Work out the finished part from the listing and answer in its coordinate system (mm). A direction names the side the tool comes from. Round coordinates to 2 decimals unless told otherwise and drop trailing zeros. Write each loop counter-clockwise with the first axis right and the second up, starting at its lowest first coordinate (ties: lowest second). Pieces come first, ordered by that corner, then holes. Notation, with made-up numbers: (89, 2) -> (105, 2) arc R9 ccw to (105, 9) -> close; hole circle Ø8 at (-10.5, 55.25). An arc over 180 degrees is marked (long way). Answer as a JSON object with one key per item and string values. Group by question number.
from build123d import *

# Parameters (mm, degrees)
SALIENTE_EXTRUIR1_DEPTH = 3.3


with BuildPart() as part:
    # Croquis1 → Saliente-Extruir1 (new body)
    with BuildSketch(Plane.XY):
        with BuildLine():
            Line((1.7, 25.8), (1.7, 35.8))
            ThreePointArc((1.7, 35.8), (4.712607831, 36.376098873), (7.730904305, 36.921609869))
            Line((7.730904305, 36.921609869), (7.730904305, 48.38))
            Line((7.730904305, 48.38), (1.7, 48.38))
            Line((1.7, 48.38), (-3.3, 48.38))
            Line((-3.3, 48.38), (-3.3, 58.38))
            Line((-3.3, 58.38), (0, 58.38))
            ThreePointArc((0, 58.38), (60, 62.669337163), (120, 58.38))
            Line((120, 58.38), (123.3, 58.38))
            Line((123.3, 58.38), (123.3, 48.38))
            Line((123.3, 48.38), (118.3, 48.38))
            Line((118.3, 48.38), (112.269095695, 48.38))
            Line((112.269095695, 48.38), (112.269095695, 36.921609869))
            ThreePointArc((112.269095695, 36.921609869), (115.287392169, 36.376098873), (118.3, 35.8))
            Line((118.3, 35.8), (118.3, 25.8))
            Line((118.3, 25.8), (123.3, 25.8))
            Line((123.3, 25.8), (123.3, 0))
            Line((123.3, 0), (120, 0))
            ThreePointArc((120, 0), (60, 35.797503597), (0, 0))
            Line((0, 0), (-3.3, 0))
            Line((-3.3, 0), (-3.3, 25.8))
            Line((-3.3, 25.8), (1.7, 25.8))
        make_face()
        with BuildLine():
            Line((17.730904305, 48.38), (17.730904305, 38.504540112))
            ThreePointArc((17.730904305, 38.504540112), (26.351558557, 39.595469902), (35, 40.438243974))
            Line((35, 40.438243974), (35, 48.38))
            Line((35, 48.38), (17.730904305, 48.38))
        make_face(mode=Mode.SUBTRACT)
        with BuildLine():
            Line((45, 48.38), (45, 41.101210552))
            ThreePointArc((45, 41.101210552), (60, 41.473490482), (75, 41.101210552))
            Line((75, 41.101210552), (75, 48.38))
            Line((75, 48.38), (45, 48.38))
        make_face(mode=Mode.SUBTRACT)
        with BuildLine():
            Line((85, 40.438243974), (85, 48.38))
            Line((85, 48.38), (102.269095695, 48.38))
            Line((102.269095695, 48.38), (102.269095695, 38.504540112))
            ThreePointArc((102.269095695, 38.504540112), (93.648441443, 39.595469902), (85, 40.438243974))
        make_face(mode=Mode.SUBTRACT)
    extrude(amount=SALIENTE_EXTRUIR1_DEPTH)


solid = part.part
1) A cutting plane is placed at B-B on z = 0.75. State how many separate pieces and enclosed holes the cut face has, plus the area to 3 significant figures.
2) A cutting plane is placed at A-A on x = 64. Determine the outline of the cut face in (y, z), plus the area to 3 significant figures.
3) Each of these flat-tipped pins is pushed along its axis until it touches: P1, Ø1.6, axis at y = 44, z = 1, coming from the +X side; P2, Ø1.6, axis at x = 92.5, z = 1.5, coming from the -Y side; P3, Ø1.5, axis at y = 35.5, z = 1.5, coming from the -X side. Where does it stop, or does it pass through?
4) A tool of negligible diameter and unlimited length cuts with its end or side. For faces 4 (the face through (2, 48.38, 2)), 5 (the face through (112.269, 43, 2)), 6 (the face through (26, 48.38, 2)), 7 (the face through (-3.3, 13, 2)), from which of +Z, -Z, +X, -X, +Y, -Y can it reach the whole face along a straight path? Write none if from no direction.
5) A cutting plane is placed at D-D on x = 39. Determine the outline of the cut face in (y, z), plus the area to 3 significant figures.
6) A cutting plane is placed at C-C on y = 15. Determine the outline of the cut face in (x, z).
7) Straight lines are drawn through the part: L1, parallel to X at y = 42.5, z = 3; L2, parallel to X at y = 41, z = 2.35; L3, parallel to X at y = 26.5, z = 1.45. For each, find the intervals that lie inside material, in ascending order.
8) For a pull along Y with two mould halves and no side action, classify faces 1 (the face through (115.245, 36.384, 1.627)), 2 (the face through (-3.3, 53, 2)), 3 (the face through (-2, 58.38, 2)) as released by +Y, released by -Y, zero draft, split by the parting line, or undercut.
Established:
{
 "1": {"separate pieces": "1", "enclosed holes": "3", "area": "3,790 mm²"},
 "2": {"outline": "(35.68, 0) -> (41.45, 0) -> (41.45, 3.3) -> (35.68, 3.3) -> close; (48.38, 0) -> (62.65, 0) -> (62.65, 3.3) -> (48.38, 3.3) -> close", "area": "66.1 mm²"},
 "3": {"P1": "stops at x = 112.27", "P2": "stops at y = 27.11", "P3": "stops at x = 1.7"},
 "4": {"face 4": "+Z, -Z, -X", "face 5": "+Z, -Z, +X", "face 6": "+Z, -Z", "face 7": "+Z, -Z, -X, +Y, -Y"},
 "5": {"outline": "(32.48, 0) -> (62.15, 0) -> (62.15, 3.3) -> (32.48, 3.3) -> close", "area": "97.9 mm²"},
 "6": {"outline": "(-3.3, 0) -> (10.97, 0) -> (10.97, 3.3) -> (-3.3, 3.3) -> close; (109.03, 0) -> (123.3, 0) -> (123.3, 3.3) -> (109.03, 3.3) -> close"},
 "7": {"L1": "x = 7.73 to 17.73, 35 to 45, 75 to 85, 102.27 to 112.27", "L2": "x = 7.73 to 17.73, 35 to 85, 102.27 to 112.27", "L3": "x = 1.7 to 25.63, 94.37 to 118.3"},
 "8": {"face 1": "undercut", "face 2": "zero draft", "face 3": "released by +Y"}
}
